Verification items for the finished model (mm, model axes). A direction names the side the tool comes from. Give positions to 0.01 mm unless a question says otherwise; leave off trailing zeros. Write each loop counter-clockwise with the first axis right and the second up, starting at its lowest first coordinate (ties: lowest second). Pieces come first, ordered by that corner, then holes. Notation, with made-up numbers: (56.25, 28) -> (115.25, 28) arc R12 ccw to (115.25, 46) -> close; hole circle Ø3 at (10.5, -23.75). An arc over 180 degrees is marked (long way). Answer as CSV lines item,"result". Start each with the question number.
1) Material ranges on L1, parallel to Y at x = -9.3, z = 0; L2, parallel to Z at x = -3.25, y = 0.5; L3, parallel to X at y = 22, z = -3, recorded low to high.
2) Mould release check, pull along Z, two halves, no side actions. Record for faces 1 (the flat face through (0, -14, -21)), 2 (the flat face through (-3, 16.2, 8.3)), 3 (the cylindrical face through (-5.44, 31.24, 6.94)): released by +Z, released by -Z, zero draft, split by the parting line, or undercut.
3) Gauge pin test, flat ends, axial feed: pin 1 Ø1.8 at (y, z) = (0, 25) entering from +X; pin 2 Ø4 at (x, z) = (-7.5, -17) entering from +Y; pin 3 Ø2 at (x, y) = (-8.5, 23.5) entering from -Z; pin 4 Ø22 at (y, z) = (-9, -3.5) entering from +X. Record the tip position at first contact, or that the pin passes through.
4) Sectioned sample at B-B on x = -4.5. Record the cut outline in (y, z), and give its area (3 significant figures).
5) Sectioned sample at A-A on x = -8. Record the cut outline in (y, z).
6) Tool access check on faces 4 (the cylindrical face through (-6.549, -12.165, 13.267)), 5 (the cylindrical face through (-8.521, -23.513, 0.195)). Record the directions out of +Z, -Z, +X, -X, +Y, -Y that give a thin tool (end or side, any length) a straight path to the whole face; none if there is none.
```python
from build123d import *

# Parameters (mm, degrees)
SKETCH1_W         = 10
SKETCH1_H         = 32
FILLET1_R         = 3
CIRPATTERN1_COUNT = 4
CHAMFER1_SIZE     = 1


with BuildPart() as part:
    # Sketch1 → Revolve1 (revolve)
    with BuildSketch(Plane.XY, mode=Mode.PRIVATE) as revolve1_sk:
        with Locations((-5, 16)):
            Rectangle(SKETCH1_W, SKETCH1_H)
    revolve(revolve1_sk.sketch.rotate(Axis((0, 0, 0), (-1, 0, 0)), 90), axis=Axis((0, 0, 0), (-1, 0, 0)))

    # Sketch2 → Cut-Revolve1 (revolve, cut)
    with BuildSketch(Plane.XY, mode=Mode.PRIVATE) as cut_revolve1_sk:
        Polygon((0, 0), (0, 25), (-3, 25), (-3, 18), (-10, 18), (-10, 0), align=None)
    revolve(cut_revolve1_sk.sketch.rotate(Axis((0, 0, 0), (-1, 0, 0)), 90), axis=Axis((0, 0, 0), (-1, 0, 0)), mode=Mode.SUBTRACT)

    # Fillet1
    fillet1_edges = [part.edges().sort_by_distance(p)[0] for p in [
        (-3, 0, 25),
    ]]
    fillet(fillet1_edges, radius=FILLET1_R - 0.0001)  # a hair under: the kernel refuses the full size

    # Sketch4 → Ø3.0mm Dowel Hole1 (revolve, cut)
    with BuildSketch(Plane(origin=(-10, 25, 0), x_dir=(0, 0, 1), z_dir=(0, 1, 0))):
        Polygon((0, 0), (0, 3.901290929), (1.5, 3), (1.5, 0), align=None)
    f_3_0mm_dowel_hole1 = revolve(axis=Axis((-16.35, 25, 0), (1, 0, 0)), mode=Mode.SUBTRACT)

    # CirPattern1: Ø3.0mm Dowel Hole1 ×4 about axis
    cirpattern1_axis = Axis((0, 0, 0), (1, 0, 0))
    for i in range(1, CIRPATTERN1_COUNT):
        add(f_3_0mm_dowel_hole1.rotate(cirpattern1_axis, i * 360 / CIRPATTERN1_COUNT), mode=Mode.SUBTRACT)

    # Chamfer1
    chamfer1_edges = [part.edges().sort_by_distance(p)[0] for p in [
        (0, 0, 32),
    ]]
    chamfer(chamfer1_edges, length=CHAMFER1_SIZE)


solid = part.part
```
Ans:
1,L1,"y = -32 to -26.5, -23.5 to -18, 18 to 23.5, 26.5 to 32"
1,L2,"z = -32 to -17.99, 17.99 to 32"
1,L3,"x = -10 to -2.99"
2,face 1,"zero draft"
2,face 2,"undercut"
2,face 3,"split by the parting line"
3,pin 1,"stops at x = 0"
3,pin 2,"stops at y = 28.27"
3,pin 3,"stops at z = -22.75"
3,pin 4,"stops at x = -3"
4,outline,"circle Ø64 at (0, 0); hole circle Ø36 at (0, 0)"
4,area,"2,200 mm²"
5,outline,"circle Ø64 at (0, 0); hole circle Ø3 at (-25, 0); hole circle Ø36 at (0, 0); hole circle Ø3 at (0, -25); hole circle Ø3 at (0, 25); hole circle Ø3 at (25, 0)"
6,face 4,"+X, -X"
6,face 5,"-X"
